Study the drawing (mm; zero at the part's minimum x, y, z) and answer. A direction names the side the tool comes from. Coordinates: 2 decimals unless noted, no trailing zeros. Order: outer loops, then holes, each group sorted by start corner. A loop starts at its lowest first (then second) coordinate and runs counter-clockwise, first axis right, second up. Notation, with made-up numbers: (15, 46) -> (56, 46) arc R16 cw to (56, 73) -> close; hole circle Ø3 at (-17.75, 7.25). An arc over 180 degrees is marked (long way). Answer as CSV lines item,"result". Start each with the question number.
Item 1: Which of the six approach directions +Z, -Z, +X, -X, +Y, -Y give full straight-line access (tool end or side, diameter ignored) to the marked faces 1, 2 and 3?
Item 2: Section A-A (y = 17) is taken. Write down the section's boundary in (x, z).
Item 3: Straight lines are drawn through the part: L1, parallel to X at y = 22.25, z = 33; L2, parallel to Z at x = 33, y = 13.75. For each, find the intervals that lie inside material, in ascending order.
Item 4: Each of these flat-tipped pins is pushed along its axis until it touches: pin 1 Ø10 at (y, z) = (7.5, 45.5) entering from +X; pin 2 Ø2 at (x, z) = (18, 35.5) entering from +Y; pin 3 Ø5 at (x, z) = (9, 41) entering from -Y. Where does it stop, or does it pass through?
Item 5: Section D-D (y = 8) is taken. Write down the section's boundary in (x, z), then the cut area to 3 significant figures.
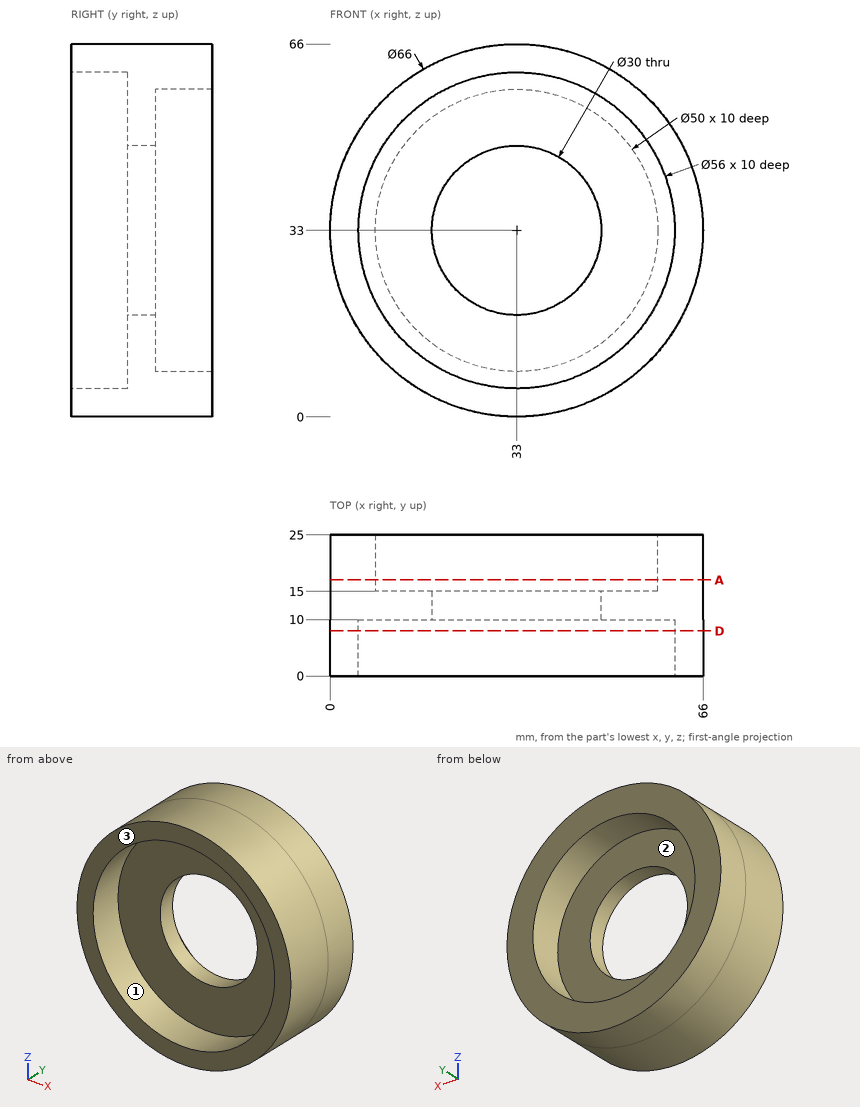
Checked values:
1,face 1,"-Y"
1,face 2,"+Y"
1,face 3,"+Z, -Z, +X, -X, -Y"
2,outline,"circle Ø66 at (33, 33); hole circle Ø50 at (33, 33)"
3,L1,"x = 0 to 8, 58 to 66"
3,L2,"z = 0 to 18, 48 to 66"
4,pin 1,"stops at x = 65.14"
4,pin 2,"stops at y = 15"
4,pin 3,"stops at y = 10"
5,outline,"circle Ø66 at (33, 33); hole circle Ø56 at (33, 33)"
5,area,"958 mm^2"
